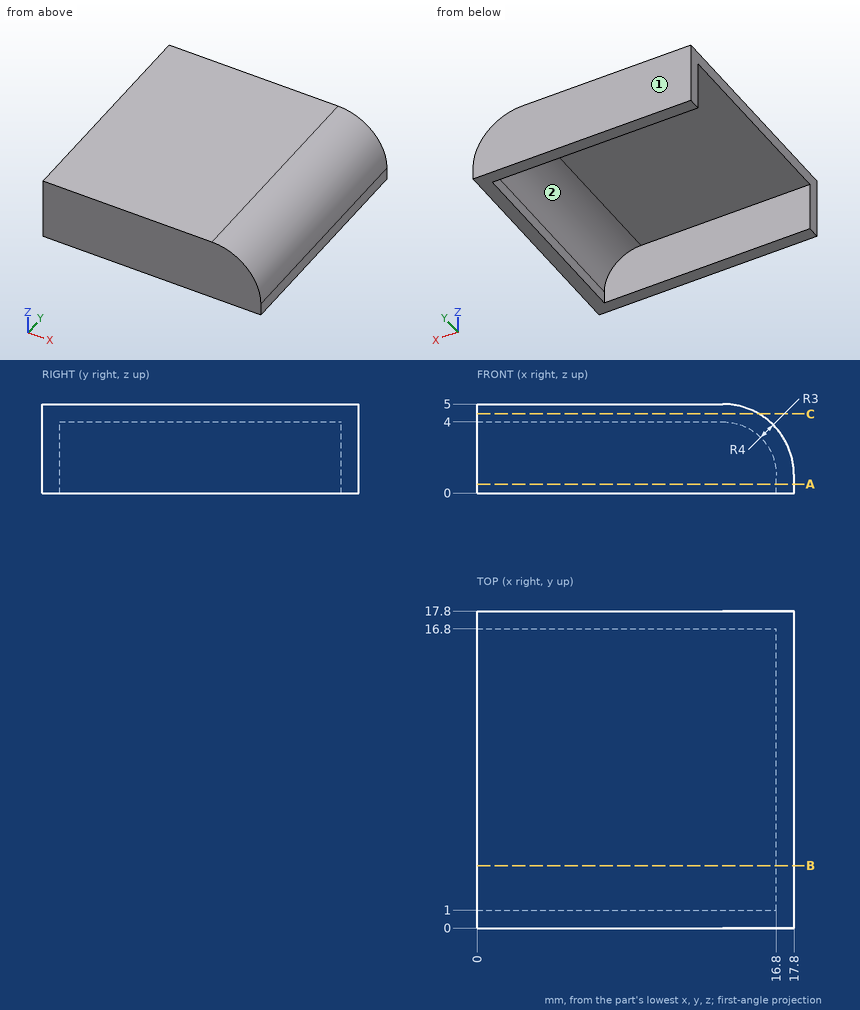
Answer from the drawing. Dimensions are ordinates in mm from the lowest x, y and z of the part. A direction names the side the tool comes from. Round coordinates to 2 decimals unless told otherwise and drop trailing zeros. Loops run counter-clockwise (first coordinate to the right, second up) from the corner with the lowest first, then second, coordinate; pieces in that order, holes last.
1) A cutting plane is placed at A-A on z = 0.5. Determine the outline of the cut face in (x, y).
Outcome:
outline: (0, 0) - (17.8, 0) - (17.8, 17.8) - (0, 17.8) - (0, 16.8) - (16.8, 16.8) - (16.8, 1) - (0, 1) - close
2) A cutting plane is placed at C-C on z = 4.45. Determine the outline of the cut face in (x, y), plus the area to 3 significant figures.
Outcome:
outline: (0, 0) - (15.82, 0) - (15.82, 17.8) - (0, 17.8) - close
area: 282 mm2
3) For the marked faces 1 and 2, determine the directions among +Z, -Z, +X, -X, +Y, -Y from which every point of the face is accessible in a straight line to the end or side of a thin tool.
Outcome:
face 1: +Z, -Z, +X, -X, +Y
face 2: -Z, -X
4) A cutting plane is placed at B-B on y = 3.5. Determine the outline of the cut face in (x, z), plus the area to 3 significant figures.
Outcome:
outline: (0, 4) - (13.8, 4) arc R3 cw to (16.8, 1) - (16.8, 0) - (17.8, 0) - (17.8, 1) arc R4 ccw to (13.8, 5) - (0, 5) - close
area: 20.3 mm2
5) Given P1, Ø0.8, axis at y = 8, z = 0.5, coming from the -X side; P2, Ø1, axis at x = 3.5, y = 16, coming from the -Z side, each flat-ended and moving along its own axis, determine where each tip first touches the part or whether it passes through.
Outcome:
P1: stops at x = 16.8
P2: stops at z = 4
6) Consider line 1 (Y direction, x = 10, z = 0.65); line 2 (Z direction, x = 7.25, y = 5.5); line 3 (X direction, y = 4, z = 0.35). Determine where each line is inside the solid, lowest interval first.
Outcome:
line 1: y = 0 to 1, 16.8 to 17.8
line 2: z = 4 to 5
line 3: x = 16.8 to 17.8
